Autodesk Inventor part; units mm, degrees
ref_plane "YZ Plane" through (0, 0, 0) normal (1, 0, 0) x (0, 1, 0)
ref_plane "XZ Plane" through (0, 0, 0) normal (0, 1, 0) x (-1, 0, 0)
ref_plane "XY Plane" through (0, 0, 0) normal (0, 0, 1) x (1, 0, 0)
sketch "스케치1" plane through (0, 0, 0) normal (0, 1, 0) x (-1, 0, 0)
  line L0 (0, 0) -> (-20, 0)
  line L1 (-20, 0) -> (-20, 27)
  line L2 (-20, 27) -> (0, 27)
  line L3 (0, 27) -> (0, 0)
  dimension "d0" = 20
  dimension "d1" = 27
extrude "돌출1" add sketch "스케치1" along normal blind 2
sketch "스케치2" plane through (0, 2, 0) normal (0, 1, 0) x (1, 0, 0)
  line L0 (20, 0) -> (0, 0)
  line L1 (0, 0) -> (0, -27)
  line L2 (0, -27) -> (20, -27)
  line L3 (20, -27) -> (20, 0)
  line L4 (20, 0) -> (0, 0)
  circle A0 centre (5, -11) radius 1.5
  circle A1 centre (15, -11) radius 1.5
  dimension "d5" = 3
  dimension "d6" = 3
  dimension "d21" = 5
  dimension "d22" = 5
  dimension "d23" = 11
  dimension "d24" = 11
extrude "돌출2" cut sketch "스케치2" against normal blind 2 contours A0 | A1
sketch "스케치3" plane through (0, 0, 0) normal (0, -1, 0) x (1, 0, 0)
  circle A0 centre (5, 11) radius 1.5
  circle A1 centre (15, 11) radius 1.5
  line L0 (0, 0) -> (20, 0)
  line L1 (20, 0) -> (20, 27)
  line L2 (20, 27) -> (0, 27)
  line L3 (0, 27) -> (0, 0)
  line L4 (5, 11) -> (5, 21)
  line L5 (15, 11) -> (15, 21)
  circle A2 centre (5, 21) radius 2.5
  circle A3 centre (15, 21) radius 2.5
  dimension "d9" = 10
  dimension "d10" = 5
  dimension "d11" = 5
extrude "돌출3" add sketch "스케치3" along normal blind 6 contours A2 | A3
sketch "스케치4" plane through (0, 2, 0) normal (0, 1, 0) x (1, 0, 0)
  circle A0 centre (5, -11) radius 1.5
  circle A1 centre (15, -11) radius 1.5
  line L0 (20, 0) -> (0, 0)
  line L1 (0, 0) -> (0, -27)
  line L2 (0, -27) -> (20, -27)
  line L3 (20, -27) -> (20, 0)
  line L4 (0, 0) -> (20, 0)
  line L5 (5, -2) -> (15, -2)
  line L6 (15, -2) -> (15, -7)
  line L7 (15, -7) -> (5, -7)
  line L8 (5, -7) -> (5, -2)
  dimension "d14" = 2
extrude "돌출4" add sketch "스케치4" along normal blind 6 contours L5 L6 L7 L8
properties part number "IR모듈"
For this review, take the finished solid that the model builds, in its own axes (mm). A direction names the side the tool comes from. Round coordinates to 2 decimals unless told otherwise and drop trailing zeros. Order: outer loops, then holes, each group sorted by start corner. A loop starts at its lowest first (then second) coordinate and runs counter-clockwise, first axis right, second up. Notation, with made-up numbers: M -23.75,18 L 30.25,18 A32 cw 30.25,50 Z; hole C 30,74 d4. An arc over 180 degrees is marked long. Use a Markdown table: item, result. Add a question column.
Item 1: Mouldability with a two-part tool opening along X and no side actions: class faces 1 (the flat face through (0, 1, 14)), 2 (the flat face through (10, 1, 27)), 3 (the flat face through (20, 1, 13)), 4 (the cylindrical face through (5.69, 1.01, 12.33)) as released by +X, released by -X, zero draft, split by the parting line, or undercut.
Item 2: Add section B-B, the plane x = 14.5. Give the boundary of the cut face in (y, z).
Item 3: Insertion check: pin 1 (5 mm diameter, centred on x = 11, y = 6, fed in from -Z); pin 2 (10 mm diameter, centred on x = 6, z = 13.5, fed in from +Y); pin 3 (3 mm diameter, centred on x = 16.5, z = 8, fed in from -Y). Each pin has a flat end and moves straight along its axis. Give the tip position at first contact, or say it passes through.
Item 4: Add section C-C, the plane z = 21. Give the boundary of the cut face in (x, y).
Item 5: Tool access review of faces 5 (the cylindrical face through (12.5, -3, 20.9)), 6 (the flat face through (5, 5, 5)), 7 (the flat face through (10, 5, 7)), 8 (the flat face through (10, 5, 2)): name each direction out of +Z, -Z, +X, -X, +Y, -Y from which nothing blocks a thin tool from reaching the whole face with its end or side.
Item 6: Add section D-D, the plane y = -3. Give the boundary of the cut face in (x, z).
Item 7: Add section A-A, the plane z = 11. Give the boundary of the cut face in (x, y).
Item 8: To check wall thickness, follow line 1 along X through (y, z) = (0.55, 11); line 2 along Z through (x, y) = (5, 1.4); line 3 along Y through (x, z) = (15.5, 19.25). State the ranges of each line that lie inside material, in increasing order.
Geometry results:
| question | item | result |
|---|---|---|
| 1 | face 1 | released by -X |
| 1 | face 2 | zero draft |
| 1 | face 3 | released by +X |
| 1 | face 4 | undercut |
| 2 | outline | M -6,18.55 L 0,18.55 L 0,12.41 L 2,12.41 L 2,27 L 0,27 L 0,23.45 L -6,23.45 Z; M 0,0 L 2,0 L 2,2 L 8,2 L 8,7 L 2,7 L 2,9.59 L 0,9.59 Z |
| 3 | pin 1 | stops at z = 2 |
| 3 | pin 2 | stops at y = 2 |
| 3 | pin 3 | stops at y = 0 |
| 4 | outline | M 0,0 L 2.5,0 L 2.5,-6 L 7.5,-6 L 7.5,0 L 12.5,0 L 12.5,-6 L 17.5,-6 L 17.5,0 L 20,0 L 20,2 L 0,2 Z |
| 5 | face 5 | -Y |
| 5 | face 6 | +Z, -Z, -X, +Y |
| 5 | face 7 | +Z, +X, -X, +Y |
| 5 | face 8 | -Z, +X, -X, +Y |
| 6 | outline | C 5,21 d5; C 15,21 d5 |
| 7 | outline | M 0,0 L 3.5,0 L 3.5,2 L 0,2 Z; M 6.5,0 L 13.5,0 L 13.5,2 L 6.5,2 Z; M 16.5,0 L 20,0 L 20,2 L 16.5,2 Z |
| 8 | line 1 | x = 0 to 3.5, 6.5 to 13.5, 16.5 to 20 |
| 8 | line 2 | z = 0 to 9.5, 12.5 to 27 |
| 8 | line 3 | y = -6 to 2 |
